Could you check a few things on this model? Use its own coordinates, in mm. A direction names the side the tool comes from. Give positions to 0.01 mm unless a question says otherwise; leave off trailing zeros. Order: outer loops, then holes, each group sorted by start corner. A loop starts at its lowest first (then second) coordinate and runs counter-clockwise, first axis right, second up.
from build123d import *

# Parameters (mm, degrees)
P_IDAT_VYSUNUT_M1_DEPTH       = 1.8
SKICA2_W                      = 30
SKICA2_H                      = 12
P_IDAT_VYSUNUT_M2_DEPTH       = 10
SKICA3_R                      = 3.5
ODEBRAT_VYSUNUT_M1_DEPTH      = 20
ODEBRAT_VYSUNUT_M2_DEPTH      = 1
ODEBRAT_VYSUNUT_M2_DEPTH_BACK = 1.5
SKICA4_W                      = 16
SKICA4_H                      = 6


with BuildPart() as part:
    # Skica1 → Přidat vysunutím1 (new body)
    with BuildSketch(Plane.XY):
        with BuildLine():
            Line((-7.5, 4.5), (7.5, 4.5))
            ThreePointArc((7.5, 4.5), (8.914213562, 3.914213562), (9.5, 2.5))
            Line((9.5, 2.5), (9.5, -2.5))
            ThreePointArc((9.5, -2.5), (8.914213562, -3.914213562), (7.5, -4.5))
            Line((7.5, -4.5), (-7.5, -4.5))
            ThreePointArc((-7.5, -4.5), (-8.914213562, -3.914213562), (-9.5, -2.5))
            Line((-9.5, -2.5), (-9.5, 2.5))
            ThreePointArc((-9.5, 2.5), (-8.914213562, 3.914213562), (-7.5, 4.5))
        make_face()
    extrude(amount=P_IDAT_VYSUNUT_M1_DEPTH)

    # Skica2 → Přidat vysunutím2 (add)
    with BuildSketch(Plane.XY.offset(1.8)):
        Rectangle(SKICA2_W, SKICA2_H)
    extrude(amount=P_IDAT_VYSUNUT_M2_DEPTH)

    # Skica3 → Odebrat vysunutím1 (cut)
    with BuildSketch(Plane(origin=(15, 0, 0), x_dir=(0, 0, -1), z_dir=(1, 0, 0))):
        with Locations((-5.8, 0)):
            Circle(SKICA3_R)
    extrude(amount=-ODEBRAT_VYSUNUT_M1_DEPTH, mode=Mode.SUBTRACT)

    # Skica4 → Odebrat vysunutím2 (cut, two sides: drawn at the far end of the back side and taken through both)
    with BuildSketch(Plane(origin=(0, 0, 1.8), x_dir=(-1, 0, 0), z_dir=(0, 0, -1)).offset(-ODEBRAT_VYSUNUT_M2_DEPTH_BACK)):
        Rectangle(SKICA4_W, SKICA4_H)
    extrude(amount=ODEBRAT_VYSUNUT_M2_DEPTH + ODEBRAT_VYSUNUT_M2_DEPTH_BACK, mode=Mode.SUBTRACT)


solid = part.part
Item 1: Imagine slicing it at A-A on x = -6.75. List the corners of the cut face in (y, z) for me, then the cut area to 3 significant figures.
Findings:
outline: (-6, 1.8) - (-4.5, 1.8) - (-4.5, 0) - (4.5, 0) - (4.5, 1.8) - (6, 1.8) - (6, 11.8) - (-6, 11.8) - close; hole (-3, 0.8) - (3, 0.8) - (3, 3.3) - (-3, 3.3) - close
area: 121 mm2
Item 2: Imagine slicing it at C-C on y = 0. List the corners of the cut face in (x, z) for me.
Findings:
outline: (-15, 1.8) - (-9.5, 1.8) - (-9.5, 0) - (9.5, 0) - (9.5, 1.8) - (15, 1.8) - (15, 2.3) - (8, 2.3) - (8, 0.8) - (-8, 0.8) - (-8, 3.3) - (-5, 3.3) - (-5, 9.3) - (15, 9.3) - (15, 11.8) - (-15, 11.8) - close
Item 3: For pin 1 (0.5 mm diameter, centred on y = -1, z = 0.5, fed in from -X); pin 2 (0.5 mm diameter, centred on x = 3, z = 1, fed in from +Y); pin 3 (0.5 mm diameter, centred on y = 1, z = 1, fed in from +X), each with a flat end and sliding along its axis, tell me the tip position at first contact or that it passes through.
Findings:
pin 1: stops at x = -9.5
pin 2: stops at y = 4.5
pin 3: stops at x = 9.5
Item 4: Please list where these lines run through material, in increasing order: line 1 along Y through (x, z) = (10.75, 5.8); line 2 along X through (y, z) = (-0.25, 2); line 3 along Z through (x, y) = (12, -5.25).
Findings:
line 1: y = -6 to -3.5, 3.5 to 6
line 2: x = -15 to -8, 8 to 15
line 3: z = 1.8 to 11.8
Item 5: Imagine slicing it at D-D on x = 10. List the corners of the cut face in (y, z) for me, then the cut area to 3 significant figures.
Findings:
outline: (-6, 1.8) - (6, 1.8) - (6, 11.8) - (-6, 11.8) - close; hole circle Ø7 at (0, 5.8)
area: 81.5 mm2
Item 6: Imagine slicing it at B-B on z = 5.8. List the corners of the cut face in (x, y) for me, then the cut area to 3 significant figures.
Findings:
outline: (-15, -6) - (15, -6) - (15, -3.5) - (-5, -3.5) - (-5, 3.5) - (15, 3.5) - (15, 6) - (-15, 6) - close
area: 220 mm2
Item 7: We'd pull the mould along Z, two halves only. Please class faces 6 (the cylindrical face through (5.14, 0.154, 9.297)), 7 (the flat face through (0, -5, 1.8)), 8 (the flat face through (9.5, 0, 1)): +Z half, -Z half, draft (parallel to the pull), parting line (faces both ways), or undercut.
Findings:
face 6: undercut
face 7: -Z half
face 8: draft
Item 8: For faces 1 (the cylindrical face through (-8.9, -3.93, 0.89)), 2 (the cylindrical face through (8.9, 3.93, 0.89)), 3 (the flat face through (-5.2, 0, 3.3)), 4 (the flat face through (-9.5, 0, 1)), 5 (the flat face through (-5, 0, 6)), which set-ups out of +Z, -Z, +X, -X, +Y, -Y let a thin tool reach every point of the face, with its end or its side?
Findings:
face 1: -Z, -X, -Y
face 2: -Z, +X, +Y
face 3: none
face 4: -Z, -X, +Y, -Y
face 5: +X
